Here's how the part is built. I have some questions about the finished solid (model axes, mm). Face numbers are marked on the shaded views. A direction names the side the tool comes from. Round coordinates to 2 decimals unless told otherwise and drop trailing zeros. Order: outer loops, then holes, each group sorted by start corner. A loop starts at its lowest first (then second) coordinate and runs counter-clockwise, first axis right, second up.
```python
from build123d import *

# Parameters (mm, degrees)
SKETCH050_W             = 144
SKETCH050_H             = 12
SKETCH050_R             = 1.9
PAD014_DEPTH            = 4
SKETCH051_R             = 4
POCKET036_DEPTH         = 2.5
FILLET012_R             = 3
SKETCH052_W             = 23
SKETCH052_H             = 9
SKETCH052_R             = 1.75
PAD015_DEPTH            = 4
BODY012_PLACEMENT_ANGLE = 270


with BuildPart() as obj1:
    # Sketch050 → Pad014 (new body)
    with BuildSketch(Plane.XZ):
        with Locations((-68, 6)):
            Rectangle(SKETCH050_W, SKETCH050_H)
        with Locations((-66, 6)):
            Circle(SKETCH050_R, mode=Mode.SUBTRACT)
        with Locations((-6, 6)):
            Circle(SKETCH050_R, mode=Mode.SUBTRACT)
        with Locations((-107.6, 6)):
            Circle(SKETCH050_R, mode=Mode.SUBTRACT)
        with Locations((-30.4, 6)):
            Circle(SKETCH050_R, mode=Mode.SUBTRACT)
        with Locations((-72, 6)):
            Circle(SKETCH050_R, mode=Mode.SUBTRACT)
        with Locations((-132, 6)):
            Circle(SKETCH050_R, mode=Mode.SUBTRACT)
    extrude(amount=PAD014_DEPTH)

    # Sketch051 (on Face11 of Pad014) → Pocket036 (cut)
    with BuildSketch(Plane(origin=(0, 0, 0), x_dir=(1, 0, 0), z_dir=(0, 1, 0))):
        with Locations((-107.6, -6)):
            Circle(SKETCH051_R)
        with Locations((-6, -6)):
            Circle(SKETCH051_R)
        with Locations((-30.4, -6)):
            Circle(SKETCH051_R)
        with Locations((-132, -6)):
            Circle(SKETCH051_R)
        with BuildLine():
            ThreePointArc((-72, -2), (-76, -6), (-72, -10))
            Line((-72, -10), (-66, -10))
            ThreePointArc((-66, -10), (-62, -6), (-66, -2))
            Line((-72, -2), (-66, -2))
        make_face()
    extrude(amount=-POCKET036_DEPTH, mode=Mode.SUBTRACT)

    # Fillet012
    fillet012_edges = [obj1.edges().sort_by_distance(p)[0] for p in [
        (4, -2, 12),
        (4, -2, 0),
    ]]
    fillet(fillet012_edges, radius=FILLET012_R)

    # Sketch052 (on Face4 of Fillet012) → Pad015 (join)
    with BuildSketch(Plane(origin=(-140, 0, 0), x_dir=(0, 0, -1), z_dir=(-1, 0, 0))):
        with Locations((-11.5, -0.5)):
            Rectangle(SKETCH052_W, SKETCH052_H)
        with Locations((-17, -0.5)):
            Circle(SKETCH052_R, mode=Mode.SUBTRACT)
    extrude(amount=-PAD015_DEPTH)


with BuildPart() as obj1_1:
    # Body012 placement: moved
    add(obj1.part.moved(Location((8.5, 121, 8))).rotate(Axis((8.5, 121, 8), (0, 0, -1)), BODY012_PLACEMENT_ANGLE))


with BuildPart() as obj1_mirrored:
    # Mirror001: instance of obj1
    add(obj1_1.part.mirror(Plane(origin=(3.1926938796, 78.5247560814, 0), x_dir=(0, 1, 0), z_dir=(-1, 0, 0))))


with BuildPart() as obj1_mirrored_1:
    # Mirror001 placement: moved
    add(obj1_mirrored.part.moved(Location((120.8, 0, 0))))


solid = obj1_mirrored_1.part
```
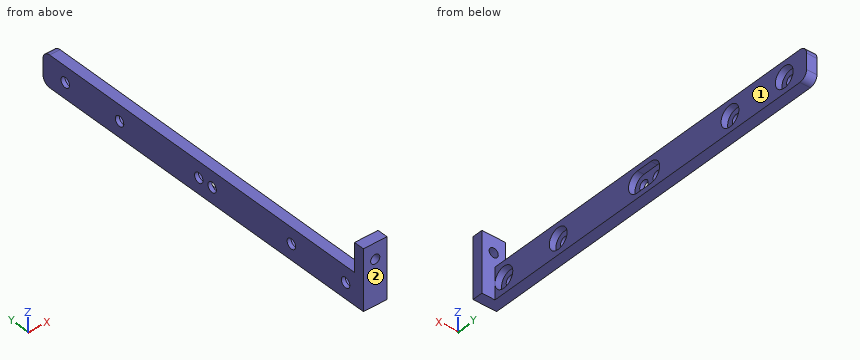
1. If we section it at B-B, the plane x = 122.5: Write out the boundary of the cut face in (y, z).
Evaluation:
outline: (-19, 8) - (-15, 8) - (-15, 31) - (-19, 31) - close
2. On a 3-axis mill with a long thin cutter (end or side, diameter ignored), from which of +Z, -Z, +X, -X, +Y, -Y can I reach the whole of each face in a straight line? I mean the marked faces 1 and 2. Say none if no direction works.
Evaluation:
face 1: +Z, -Z, +X, +Y
face 2: +Z, -Z, +X, -X, -Y
3. If we section it at C-C, the plane y = 30.5: Write out the boundary of the cut face in (x, z), and give its area (3 significant figures).
Evaluation:
outline: (114.69, 8) - (118.69, 8) - (118.69, 20) - (114.69, 20) - close
area: 48.0 mm2
4. I need wall thicknesses on probe 1 along Z at (x, y) = (116.9, 115); probe 2 along Z at (x, y) = (115.35, 115); probe 3 along Y at (x, z) = (118.5, 14.5). Which ranges of each line are inside material? Lowest first, please.
Evaluation:
probe 1: z = 8 to 10, 18 to 20
probe 2: z = 8 to 12.1, 15.9 to 20
probe 3: y = -19 to -14.97, -7.03 to 9.43, 17.37 to 45.03, 58.97 to 86.63, 94.57 to 111.03, 118.97 to 125
5. I'm going to push flat-ended pins straight in: P1, Ø4, axis at y = -10, z = 13.5, coming from the +X side; P2, Ø4.5, axis at x = 116, y = 64, coming from the +Z side; P3, Ø4.5, axis at x = 119.19, z = 25, coming from the +Y side. Where does each tip first touch, or does it pass through?
Evaluation:
P1: stops at x = 116.19
P2: stops at z = 20
P3: stops at y = -15
6. If we section it at A-A, the plane y = 13.4: Write out the boundary of the cut face in (x, z).
Evaluation:
outline: (114.69, 8) - (118.69, 8) - (118.69, 10) - (116.19, 10) - (116.19, 12.1) - (114.69, 12.1) - close; (114.69, 15.9) - (116.19, 15.9) - (116.19, 18) - (118.69, 18) - (118.69, 20) - (114.69, 20) - close
